Autodesk Inventor part; units mm, degrees
ref_plane "Plano de trabajo1" through (0, 0, 0) normal (0, 0, 1) x (1, 0, 0)
ref_plane "YZ Plane" through (0, 0, 0) normal (1, 0, 0) x (0, 1, 0)
ref_plane "XZ Plane" through (0, 0, 0) normal (0, 1, 0) x (-1, 0, 0)
sketch "Boceto1" plane through (0, 0, 0) normal (0, 1, 0) x (-1, 0, 0)
  circle A0 centre (0, 0) radius 10.95
  dimension "d0" = 21.9
extrude "Extrusión1" add sketch "Boceto1" along normal blind 146.5
sketch "Boceto2" plane through (0, 0, 0) normal (0, -1, 0) x (1, 0, 0)
  circle A0 centre (3.4074, 3.75) radius 3
  circle A1 centre (3.4074, -3.75) radius 3
  circle A2 centre (-4.9805, 0) radius 3.5
  point P0 (0, 0)
  dimension "d3" = 6
  dimension "d4" = 6
  dimension "d5" = 7
  dimension "d" = 7.5
  dimension "d7" = 3.75
extrude "Extrusión2" cut sketch "Boceto2" against normal blind 40.5
sketch "Boceto4" plane through (0, 0, 0) normal (0, -1, 0) x (1, 0, 0)
  circle A0 centre (0, 0) radius 10.95
  circle A1 centre (0, 0) radius 11
  dimension "d10" = 22
extrude "Extrusión3" add sketch "Boceto4" against normal blind 41.5
sketch "Boceto5" plane through (0, 146.5, 0) normal (0, 1, 0) x (1, 0, 0)
  circle A0 centre (0, 0) radius 10.95
extrude "Extrusión4" cut sketch "Boceto5" against normal blind 105
ref_plane "Plano de trabajo1" through (0, 0, 0) normal (0, 0, 1) x (1, 0, 0)
sketch "Boceto6" plane through (0, 0, 0) normal (0, 0, 1) x (1, 0, 0)
  circle A0 centre (5.8998, 33.6799) radius 3
  point P0 (0, 0)
  dimension "d16" = 6
extrude "Extrusión5" cut sketch "Boceto6" along normal mid plane 22
properties part number "W520inferior"
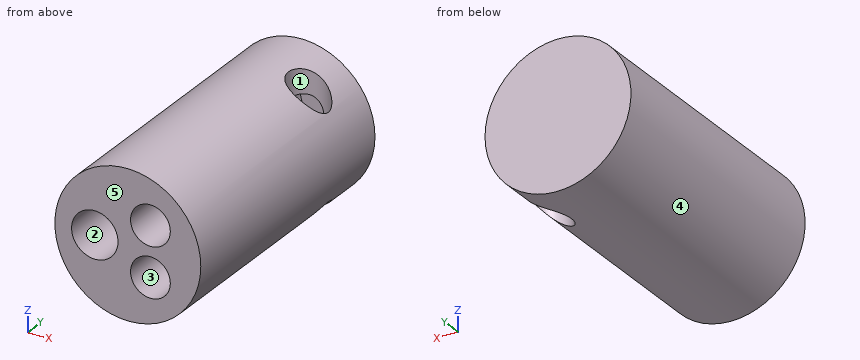
Can you work these out from the model? Positions are in its coordinate system, mm. Face numbers are marked on the shaded views. A direction names the side the tool comes from. Give positions to 0.01 mm unless a question says otherwise; leave off trailing zeros. Loops run counter-clockwise (first coordinate to the right, second up) from the corner with the lowest first, then second, coordinate; pieces in that order, holes last. Notation, with made-up numbers: M 5,7.25 L 23,7.25 A24 ccw 23,36.25 Z; hole C -36.75,-31 d3. An arc over 180 degrees is marked long. One line per item, written item: value.
(1) Suppose I cut it at D-D on y = 17.5. List the corners of the cut face in (x, z) for me.
Returned:
outline: C 0,0 d22; hole C -4.98,0 d7; hole C 3.41,-3.75 d6; hole C 3.41,3.75 d6
(2) I need wall thicknesses on line 1 (Z direction, x = 2.75, y = 38); line 2 (X direction, y = 2.5, z = -2.25); line 3 (Z direction, x = 6, y = 27). Which ranges of each line are inside material? Lowest first, please.
Returned:
line 1: -10.65 to -6.68, -0.82 to 0.82, 6.68 to 10.65
line 2: -10.77 to -7.66, -2.3 to 0.81, 6.01 to 10.77
line 3: -9.22 to -5.26, -2.24 to 2.24, 5.26 to 9.22
(3) We'd pull the mould along Z, two halves only. Please class the marked faces 3, 4 and 5: released by +Z, released by -Z, zero draft, split by the parting line, or undercut.
Returned:
face 3: undercut
face 4: split by the parting line
face 5: zero draft
(4) Will these pins go through, and if not, where does the flat tip stop? pin 1 (1.8 mm diameter, centred on x = 3.5, z = 5, fed in from -Y); pin 2 (3 mm diameter, centred on x = 7.5, y = 31, fed in from -Z); pin 3 (1.5 mm diameter, centred on y = 11.5, z = 1, fed in from -X).
Returned:
pin 1: y = 40.5
pin 2: z = -9.2
pin 3: x = -11
(5) Suppose I cut it at B-B on y = 35.5. Count the separate pieces of the cut face and the enclosed holes in it, plus the area to 3 significant figures.
Returned:
separate pieces: 2
enclosed holes: 1
area: 225 mm^2
(6) Which directions (+Z, -Z, +X, -X, +Y, -Y) give clear straight access to the entire face, cutting with the end or side of a thin tool? Please do the marked faces 1 and 2.
Returned:
face 1: +Z, -Z
face 2: -Y
(7) Suppose I cut it at A-A on x = 8.25. List the corners of the cut face in (y, z) for me, plus the area to 3 significant figures.
Returned:
outline: M 0,-7.28 L 31.82,-7.28 L 31.82,7.28 L 0,7.28 Z; M 35.54,-7.28 L 41.5,-7.28 L 41.5,7.28 L 35.54,7.28 Z
area: 550 mm^2
(8) Suppose I cut it at C-C on z = 0. List the corners of the cut face in (x, y) for me, plus the area to 3 significant figures.
Returned:
outline: M -11,0 L -8.48,0 L -8.48,40.5 L -1.48,40.5 L -1.48,0 L 11,0 L 11,41.5 L -11,41.5 Z; hole C 5.9,33.68 d6
area: 601 mm^2
